```python
from build123d import *

# Parameters (mm, degrees)
F1_DEPTH = 7.62


with BuildPart() as f1:
    # F0 (on Top) → F1 (new body)
    with BuildSketch(Plane.XY):
        Polygon((6.422935, 38.444217), (-14.166216, 38.444217), (-21.403519, 31.57974), (-5.64046, 31.57974), (-15.981315, 18.460336), (-68.928845, 60.194146), (-93.437128, 51.977817), (-72.384275, 25.243798), (-64.864993, 29.134912), (-70.054352, 22.652369), (-48.670258, -1.8672), (-40.059935, 3.577625), (-46.473149, -5.455938), (-30.269377, -22.767998), (-19.772258, -13.421346), (-22.834825, -34.648044), (0, -57.534426), (23.207549, -34.379158), (19.991519, -13.223941), (30.720653, -22.767998), (46.702418, -4.801791), (40.234059, 3.875277), (49.077254, -1.836646), (70.586123, 22.652369), (64.496264, 29.908372), (72.788842, 25.243798), (93.672454, 51.977817), (68.720646, 59.903685), (18.547656, 20.028364), align=None)
    extrude(amount=F1_DEPTH)


solid = f1.part
```
For this review, take the finished solid that the model builds, in its own axes (mm). A direction names the side the tool comes from. Round coordinates to 2 decimals unless told otherwise and drop trailing zeros. Loops run counter-clockwise (first coordinate to the right, second up) from the corner with the lowest first, then second, coordinate; pieces in that order, holes last.
Q1. Add section D-D on x = 8.5. Write out the cut boundary in (y, z).
Result sheet:
outline: (-49.05, 0) - (35.29, 0) - (35.29, 7.62) - (-49.05, 7.62) - close
Q2. Mouldability with a two-part tool opening along X and no side actions: class faces 1 (the face through (43.51, -0.52, 3.76)), 2 (the face through (-81.011, 56.143, 3.757)), 3 (the face through (-68.68, 27.16, 3.76)), 4 (the face through (-1, 15, 7.62)) as +X half, -X half, draft (parallel to the pull), parting line (faces both ways), or undercut.
Result sheet:
face 1: undercut
face 2: -X half
face 3: undercut
face 4: draft
Q3. Machinability: for faces 5 (the face through (-4, 38.444, 4)), 6 (the face through (21.622, -23.95, 3.757)), 7 (the face through (-11.58, -45.93, 3.76)), which of the approach directions +Z, -Z, +X, -X, +Y, -Y give a long, thin tool a straight path to every point of the face, cutting with its end or side? Answer none if there is none.
Result sheet:
face 5: +Z, -Z, +Y
face 6: +Z, -Z
face 7: +Z, -Z, -X, -Y
Q4. Add section A-A on y = 43. Write out the cut boundary in (x, z).
Result sheet:
outline: (-86.37, 0) - (-47.11, 0) - (-47.11, 7.62) - (-86.37, 7.62) - close; (47.45, 0) - (86.66, 0) - (86.66, 7.62) - (47.45, 7.62) - close
Q5. Add section C-C on y = -19.5. Write out the cut boundary in (x, z).
Result sheet:
outline: (-33.33, 0) - (-26.6, 0) - (-26.6, 7.62) - (-33.33, 7.62) - close; (-20.65, 0) - (20.95, 0) - (20.95, 7.62) - (-20.65, 7.62) - close; (27.05, 0) - (33.63, 0) - (33.63, 7.62) - (27.05, 7.62) - close
Q6. Insertion check: pin 1 Ø4 at (y, z) = (-3, 6.5) entering from -X; pin 2 Ø3 at (y, z) = (40.5, 6.5) entering from +X; pin 3 Ø3 at (x, z) = (-29, 2.5) entering from +Y. Each pin has a flat end and moves straight along its axis. Give the tip position at first contact, or say it passes through.
Result sheet:
pin 1: stops at x = -49.43
pin 2: stops at x = 85.88
pin 3: stops at y = 29.9
Q7. To check wall thickness, follow line 1 along X through (y, z) = (2.5, 5.5); line 2 along X through (y, z) = (-15, 3.5); line 3 along X through (y, z) = (28, 4.5). State the ranges of each line that lie inside material, in increasing order.
Result sheet:
line 1: x = -52.48 to -41.76, -40.82 to 41.26, 42.36 to 52.89
line 2: x = -37.54 to -21.55, -20 to 20.26, 21.99 to 37.63
line 3: x = -74.55 to -67.06, -65.77 to -28.08, -8.46 to 13.3, 28.58 to 66.1, 67.89 to 74.94
